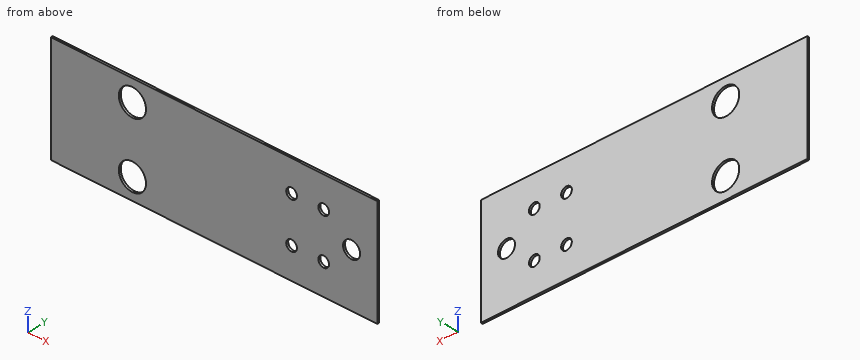
from build123d import *

# Parameters (mm, degrees)
ESQUISSE1_W             = 152.4
ESQUISSE1_H             = 50.8
BOSS_EXTRU_1_DEPTH      = 1
ESQUISSE2_R             = 6.35
ENL_V_MAT_EXTRU_1_DEPTH = 1
ESQUISSE3_R             = 2.5
ENL_V_MAT_EXTRU_2_DEPTH = 1
ESQUISSE4_R             = 3.96875
ENL_V_MAT_EXTRU_3_DEPTH = 1


with BuildPart() as part:
    # Esquisse1 → Boss.-Extru.1 (new body)
    with BuildSketch(Plane(origin=(0, 0, 0), x_dir=(1, 0, 0), z_dir=(0, 1, 0))):
        Rectangle(ESQUISSE1_W, ESQUISSE1_H)
    extrude(amount=BOSS_EXTRU_1_DEPTH)

    # Esquisse2 → Enlèv. mat.-Extru.1 (cut)
    with BuildSketch(Plane(origin=(0, 1, 0), x_dir=(1, 0, 0), z_dir=(0, 1, 0))):
        with Locations((-38.1, 15.4)):
            Circle(ESQUISSE2_R)
        with Locations((-38.1, -15.4)):
            Circle(ESQUISSE2_R)
    extrude(amount=-ENL_V_MAT_EXTRU_1_DEPTH, mode=Mode.SUBTRACT)

    # Esquisse3 → Enlèv. mat.-Extru.2 (cut)
    with BuildSketch(Plane(origin=(0, 1, 0), x_dir=(1, 0, 0), z_dir=(0, 1, 0))):
        with Locations((51.2, 10.775)):
            Circle(ESQUISSE3_R)
        with Locations((36.2, 10.775)):
            Circle(ESQUISSE3_R)
        with Locations((36.2, -10.775)):
            Circle(ESQUISSE3_R)
        with Locations((51.2, -10.775)):
            Circle(ESQUISSE3_R)
    extrude(amount=-ENL_V_MAT_EXTRU_2_DEPTH, mode=Mode.SUBTRACT)

    # Esquisse4 → Enlèv. mat.-Extru.3 (cut)
    with BuildSketch(Plane(origin=(0, 1, 0), x_dir=(1, 0, 0), z_dir=(0, 1, 0))):
        with Locations((64.2, 0)):
            Circle(ESQUISSE4_R)
    extrude(amount=-ENL_V_MAT_EXTRU_3_DEPTH, mode=Mode.SUBTRACT)


solid = part.part
Geometry: final body of the model. Coordinates: model frame, mm. Coordinates: 2 decimals unless noted, no trailing zeros. Order: outer loops, then holes, each group sorted by start corner. A loop starts at its lowest first (then second) coordinate and runs counter-clockwise, first axis right, second up.
(1) Material intervals for probe 1 along Z at (x, y) = (-38.1, 0.4); probe 2 along Z at (x, y) = (51.2, 0.6) (3 decimals); probe 3 along X at (y, z) = (0.35, 15.4), sorted ascending.
(2) First-contact query: pin 1 (8 mm diameter, centred on x = -38, z = 18.5, fed in from -Y); pin 2 (11.5 mm diameter, centred on x = -38.1, z = 15.4, fed in from -Y). Flat tips, straight axial feed; report the tip coordinate or a pass-through.
(3) Section query D-D (y = 0.2). State how many separate pieces and enclosed holes the cut face has, plus the area to 3 significant figures.
(4) Section query C-C (z = 15.4). Return the cut outline in (x, y).
(5) Section query A-A (x = 64.2). Return the cut outline in (y, z).
(6) Section query B-B (x = -38.1). Return the cut outline in (y, z), plus the area to 3 significant figures.
Solution:
1. probe 1: z = -25.4 to -21.75, -9.05 to 9.05, 21.75 to 25.4
1. probe 2: z = -25.4 to -13.275, -8.275 to 8.275, 13.275 to 25.4
1. probe 3: x = -76.2 to -44.45, -31.75 to 76.2
2. pin 1: stops at y = 0
2. pin 2: passes through
3. separate pieces: 1
3. enclosed holes: 7
3. area: 7,360 mm2
4. outline: (-76.2, 0) - (-44.45, 0) - (-44.45, 1) - (-76.2, 1) - close; (-31.75, 0) - (76.2, 0) - (76.2, 1) - (-31.75, 1) - close
5. outline: (0, -25.4) - (1, -25.4) - (1, -3.97) - (0, -3.97) - close; (0, 3.97) - (1, 3.97) - (1, 25.4) - (0, 25.4) - close
6. outline: (0, -25.4) - (1, -25.4) - (1, -21.75) - (0, -21.75) - close; (0, -9.05) - (1, -9.05) - (1, 9.05) - (0, 9.05) - close; (0, 21.75) - (1, 21.75) - (1, 25.4) - (0, 25.4) - close
6. area: 25.4 mm2
